Geometry check sheet. Reference: the model listing, model coordinates, mm. Face numbers are marked on the shaded views. A direction names the side the tool comes from. Give positions to 0.01 mm unless a question says otherwise; leave off trailing zeros. Write each loop counter-clockwise with the first axis right and the second up, starting at its lowest first coordinate (ties: lowest second). Pieces come first, ordered by that corner, then holes. Notation, with made-up numbers: (-32.75, 7.5) -> (24.25, 7.5) arc R12 ccw to (24.25, 27.5) -> close; hole circle Ø9 at (29.5, 6). An arc over 180 degrees is marked (long way). One line per item, written item: value.
from build123d import *

# Parameters (mm, degrees)
SKETCH067_R          = 2.25
PAD043_DEPTH         = 15
SKETCH068_R          = 10
PAD044_DEPTH         = 5
SKETCH069_W          = 22.6375
SKETCH069_H          = 11
POCKET022_DEPTH      = 12.001
POCKET022_DEPTH_BACK = 12.001


with BuildPart() as part:
    # Sketch067 → Pad043 (new body)
    with BuildSketch(Plane.XY):
        with BuildLine():
            ThreePointArc((10, 21.26617), (0, 23.5), (-10, 21.26617))
            Line((-10, 21.26617), (-10, -21.26617))
            ThreePointArc((-10, -21.26617), (0, -23.5), (10, -21.26617))
            Line((10, -21.26617), (10, 21.26617))
        make_face()
        with Locations((0, 19)):
            Circle(SKETCH067_R, mode=Mode.SUBTRACT)
        with Locations((0, -19)):
            Circle(SKETCH067_R, mode=Mode.SUBTRACT)
    extrude(amount=PAD043_DEPTH)

    # Sketch068 → Pad044 (join, symmetric)
    with BuildSketch(Plane.XZ):
        with BuildLine():
            ThreePointArc((11.756992, 23.597266), (0, 38), (-11.756992, 23.597266))
            Line((-11.756992, 23.597266), (-10, 15))
            Line((10, 15), (-10, 15))
            Line((11.756992, 23.597266), (10, 15))
        make_face()
        with Locations((0, 26)):
            Circle(SKETCH068_R, mode=Mode.SUBTRACT)
    extrude(amount=PAD044_DEPTH, both=True)

    # Sketch069 → Pocket022 (cut, two sides)
    with BuildSketch(Plane.YZ) as pocket022_sk:
        with Locations((0, 5.5)):
            Rectangle(SKETCH069_W, SKETCH069_H)
    extrude(amount=-POCKET022_DEPTH, mode=Mode.SUBTRACT)
    extrude(pocket022_sk.sketch, amount=POCKET022_DEPTH_BACK, mode=Mode.SUBTRACT)


solid = part.part
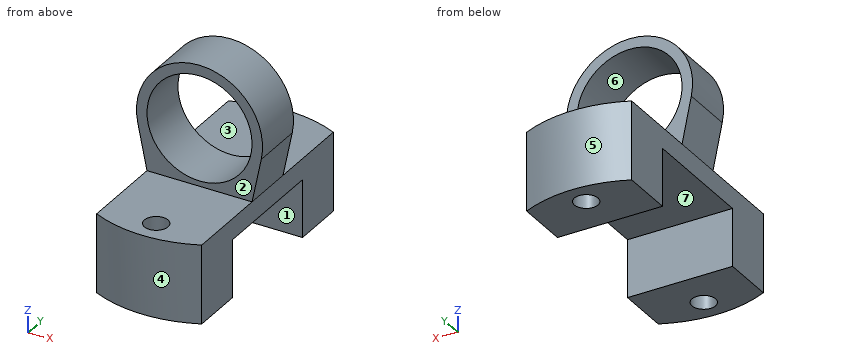
1) Sectioned sample at B-B on y = -19. Record the cut outline in (x, z), plus the area to 4 significant figures.
Verdict:
outline: (-10, 0) -> (-2.25, 0) -> (-2.25, 15) -> (-10, 15) -> close; (2.25, 0) -> (10, 0) -> (10, 15) -> (2.25, 15) -> close
area: 232.5 mm^2
2) Sectioned sample at A-A on x = 0. Record the cut outline in (y, z).
Verdict:
outline: (-23.5, 0) -> (-21.25, 0) -> (-21.25, 15) -> (-23.5, 15) -> close; (-16.75, 0) -> (-11.32, 0) -> (-11.32, 11) -> (11.32, 11) -> (11.32, 0) -> (16.75, 0) -> (16.75, 15) -> (5, 15) -> (5, 16) -> (-5, 16) -> (-5, 15) -> (-16.75, 15) -> close; (-5, 36) -> (5, 36) -> (5, 38) -> (-5, 38) -> close; (21.25, 0) -> (23.5, 0) -> (23.5, 15) -> (21.25, 15) -> close
3) Scan lines: probe 1 along Z at (x, y) = (-9.5, 15); probe 2 along Z at (x, y) = (9.25, -7.5); probe 3 along Z at (x, y) = (3.5, -3). Record each from-to range of solid material in increasing order.
Verdict:
probe 1: 0 to 15
probe 2: 11 to 15
probe 3: 11 to 16.63, 35.37 to 37.48
4) Sectioned sample at C-C on z = 26. Record the cut outline in (x, y), plus the area to 3 significant figures.
Verdict:
outline: (-12, -5) -> (-10, -5) -> (-10, 5) -> (-12, 5) -> close; (10, -5) -> (12, -5) -> (12, 5) -> (10, 5) -> close
area: 40.0 mm^2
5) Depth check by flat-ended pin: pin 1 Ø1.5 at (y, z) = (-14.5, 9) entering from +X; pin 2 Ø1.5 at (x, y) = (3.5, -3) entering from +Z; pin 3 Ø2 at (y, z) = (-6.5, 22.5) entering from -X; pin 4 Ø5 at (x, y) = (0, -19) entering from +Z. Enter the tip coordinate at first touch or a pass-through.
Verdict:
pin 1: x = 10
pin 2: z = 37.68
pin 3: through
pin 4: z = 15
6) Tool access check on the marked faces 1, 2, 3 and 4. Record the directions out of +Z, -Z, +X, -X, +Y, -Y that give a thin tool (end or side, any length) a straight path to the whole face; none if there is none.
Verdict:
face 1: -Z, +X, -X
face 2: +Z, +X, -X, -Y
face 3: +Z, +X, -X, +Y
face 4: +Z, -Z, -Y
7) Sectioned sample at D-D on y = 1. Record the cut outline in (x, z).
Verdict:
outline: (-11.76, 23.6) -> (-10, 15) -> (-10, 11) -> (10, 11) -> (10, 15) -> (11.76, 23.6) arc R12 ccw (long way) to start; hole circle Ø20 at (0, 26)
8) Mould release check, pull along Y, two halves, no side actions. Record for the marked faces 5, 6 and 7: released by +Y, released by -Y, zero draft, split by the parting line, or undercut.
Verdict:
face 5: released by +Y
face 6: zero draft
face 7: undercut
